The figure shows three views and two pictorial views of one solid part (mm, origin at its lowest corner). Answer the questions. A direction names the side the tool comes from. Coordinates: 2 decimals unless noted, no trailing zeros. Order: outer loops, then holes, each group sorted by start corner. A loop starts at its lowest first (then second) coordinate and runs counter-clockwise, first axis right, second up. Notation, with made-up numbers: (29, 39) - (84, 39) arc R29 cw to (84, 66) - close; hole circle Ø7 at (88, -30). An arc over 180 degrees is marked (long way). Answer as a JSON object with one key per item and string values. Group by question number.
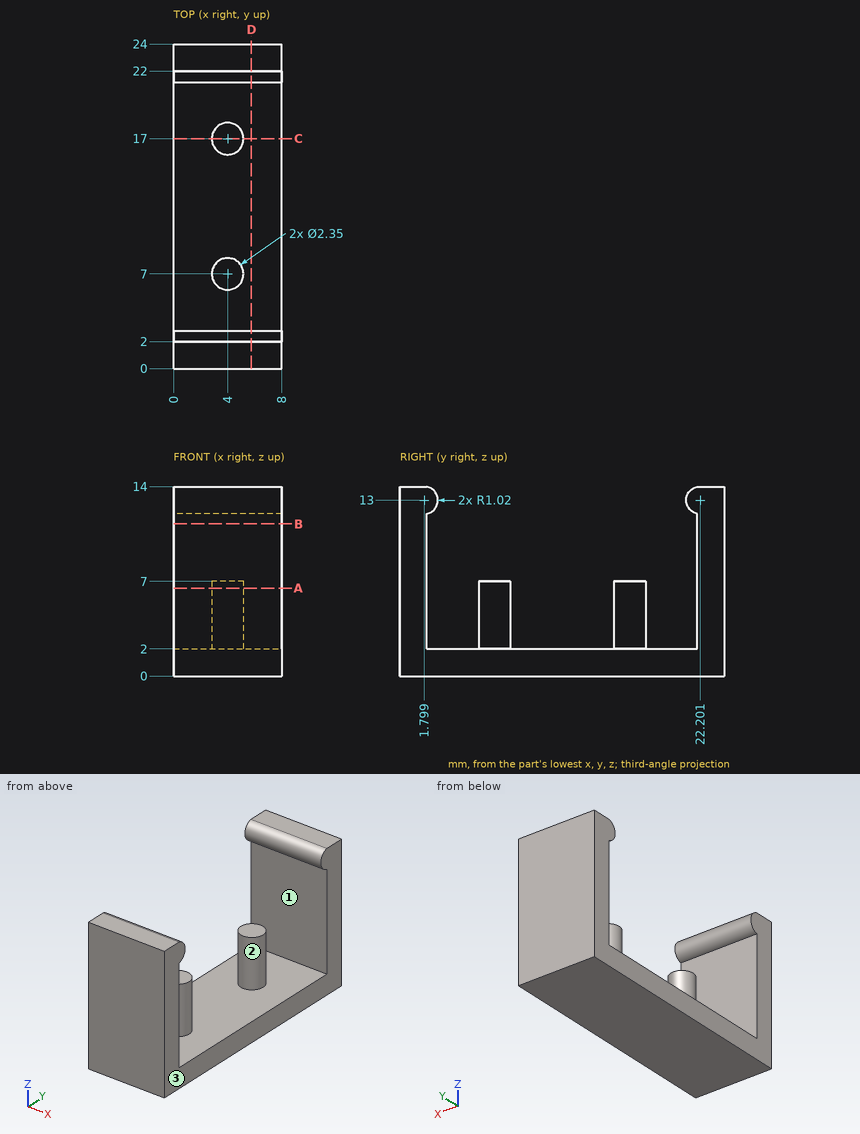
1. A cutting plane is placed at D-D on x = 5.75. Write down the section's boundary in (y, z).
2. For the marked faces 1, 2 and 3, determine the directions among +Z, -Z, +X, -X, +Y, -Y from which every point of the face is accessible in a straight line to the end or side of a thin tool.
3. A cutting plane is placed at B-B on z = 11.25. Write down the section's boundary in (x, y).
4. Given pin 1 (2.5 mm diameter, centred on x = 3.5, y = 17, fed in from +Z); pin 2 (5 mm diameter, centred on y = 13.5, z = 6, fed in from +X), each flat-ended and moving along its own axis, determine where each tip first touches the part or whether it passes through.
5. A cutting plane is placed at C-C on y = 17. Write down the section's boundary in (x, z) (3 decimals).
6. A cutting plane is placed at A-A on z = 6.5. Write down the section's boundary in (x, y) (3 decimals).
7. Straight lines are drawn through the part: L1, parallel to Y at x = 2.75, z = 3.25; L2, parallel to Z at x = 1.5, y = 16.75; L3, parallel to Y at x = 3.75, z = 12.5. For each, find the intervals that lie inside material, in ascending order.
Derived:
{
 "1": {"outline": "(0, 0) - (24, 0) - (24, 14) - (22, 14) arc R1.02 ccw to (22, 12) - (22, 2) - (2, 2) - (2, 12) arc R1.02 ccw to (2, 14) - (0, 14) - close"},
 "2": {"face 1": "+X, -X", "face 2": "+Z", "face 3": "+Z, -Z, +X, +Y, -Y"},
 "3": {"outline": "(0, 0) - (8, 0) - (8, 2) - (0, 2) - close; (0, 22) - (8, 22) - (8, 24) - (0, 24) - close"},
 "4": {"pin 1": "stops at z = 7", "pin 2": "stops at x = 4.62"},
 "5": {"outline": "(0, 0) - (8, 0) - (8, 2) - (5.175, 2) - (5.175, 7) - (2.825, 7) - (2.825, 2) - (0, 2) - close"},
 "6": {"outline": "(0, 0) - (8, 0) - (8, 2) - (0, 2) - close; (0, 22) - (8, 22) - (8, 24) - (0, 24) - close; circle Ø2.35 at (4, 7); circle Ø2.35 at (4, 17)"},
 "7": {"L1": "y = 0 to 2, 22 to 24", "L2": "z = 0 to 2", "L3": "y = 0 to 2.69, 21.31 to 24"}
}
